from build123d import *

# Parameters (mm, degrees)
F0_W     = 25
F0_H     = 10
F1_DEPTH = 5
F2_R     = 1.4
F3_DEPTH = 25
F2_W     = 8
F2_H     = 10
F4_DEPTH = 7
F5_R     = 1.4
F6_DEPTH = 25
F2_R_2   = 2.5
F7_DEPTH = 2.5


with BuildPart() as f1:
    # F0 (on Top) → F1 (new body)
    with BuildSketch(Plane.XY):
        Rectangle(F0_W, F0_H)
    extrude(amount=F1_DEPTH)

    # F2 (on face) → F3 (cut)
    with BuildSketch(Plane.XY.offset(5)):
        with Locations((-9.5, 0.5)):
            Circle(F2_R)
    extrude(amount=-F3_DEPTH, mode=Mode.SUBTRACT)

    # F2 (on face) → F4 (join)
    with BuildSketch(Plane.XY.offset(5)):
        with Locations((8.5, 0)):
            Rectangle(F2_W, F2_H)
    extrude(amount=F4_DEPTH)

    # F5 (on face) → F6 (cut)
    with BuildSketch(Plane(origin=(4.5, 0, 0), x_dir=(0, -1, 0), z_dir=(-1, 0, 0))):
        with Locations((-2.647824, 9.4)):
            Circle(F5_R)
    extrude(amount=-F6_DEPTH, mode=Mode.SUBTRACT)

    # F2 (on face) → F7 (cut)
    with BuildSketch(Plane.XY.offset(5)):
        with Locations((-9.5, 0.5)):
            Circle(F2_R_2)
        with Locations((-9.5, 0.5)):
            Circle(F2_R, mode=Mode.SUBTRACT)
    extrude(amount=-F7_DEPTH, mode=Mode.SUBTRACT)


solid = f1.part
Geometry check sheet. Reference: the model listing, model coordinates, mm. A direction names the side the tool comes from. Round coordinates to 2 decimals unless told otherwise and drop trailing zeros. Write each loop counter-clockwise with the first axis right and the second up, starting at its lowest first coordinate (ties: lowest second). Pieces come first, ordered by that corner, then holes. Notation, with made-up numbers: (-39, -3) -> (-9, -3) arc R20 ccw to (-9, 32) -> close; hole circle Ø4 at (72, 84). An arc over 180 degrees is marked (long way). One line per item, written item: value. Start each with the question number.
(1) Cross-section at B-B, the plane z = 1.5. Record the cut outline in (x, y), and give its area (3 significant figures).
(2) Go/stop test with flat-tipped pins: pin 1 Ø4.5 at (y, z) = (2.65, 9.4) entering from -X; pin 2 Ø2 at (x, y) = (-9.5, 0.5) entering from +Z; pin 3 Ø5.5 at (x, y) = (-9.5, 1) entering from +Z. Record where each tip stops, or that it passes through.
(3) Cross-section at C-C, the plane x = 7.5. Record the cut outline in (y, z).
(4) Draft check along Y on faces 4 (the cylindrical face through (8.444, 1.312, 9.821)), 5 (the flat face through (12.5, 0, 6)), 6 (the flat face through (2.6, 5, 4.6)). Enter one of: +Y half, -Y half, draft (parallel to the pull), parting line (faces both ways), or undercut.
(5) Scan lines: line 1 (Y direction, x = -9.5, z = 4.3); line 2 (X direction, y = 4, z = 8.5); line 3 (Z direction, x = 3.5, y = 1). Record each from-to range of solid material in increasing order. Write a range as [from, to].
(6) Cross-section at D-D, the plane z = 9.4. Record the cut outline in (x, y).
(7) Cross-section at A-A, the plane y = 0.5. Record the cut outline in (x, z), and give its area (4 significant figures).
(8) Access from +Z, -Z, +X, -X, +Y, -Y to the whole of each face (thin tool, end or side, straight path). Record for faces 1 (the flat face through (-4, 0, 5)), 2 (the flat face through (-8, -1, 2.5)), 3 (the flat face through (8, 0, 12)).
Answer:
1. outline: (-12.5, -5) -> (12.5, -5) -> (12.5, 5) -> (-12.5, 5) -> close; hole circle Ø2.8 at (-9.5, 0.5)
1. area: 244 mm²
2. pin 1: x = 4.5
2. pin 2: through
2. pin 3: z = 5
3. outline: (-5, 0) -> (5, 0) -> (5, 12) -> (-5, 12) -> close; hole circle Ø2.8 at (2.65, 9.4)
4. face 4: undercut
4. face 5: draft
4. face 6: +Y half
5. line 1: [-5, -2], [3, 5]
5. line 2: [4.5, 12.5]
5. line 3: [0, 5]
6. outline: (4.5, -5) -> (12.5, -5) -> (12.5, 1.25) -> (4.5, 1.25) -> close; (4.5, 4.05) -> (12.5, 4.05) -> (12.5, 5) -> (4.5, 5) -> close
7. outline: (-12.5, 0) -> (-10.9, 0) -> (-10.9, 2.5) -> (-12, 2.5) -> (-12, 5) -> (-12.5, 5) -> close; (-8.1, 0) -> (12.5, 0) -> (12.5, 12) -> (4.5, 12) -> (4.5, 5) -> (-7, 5) -> (-7, 2.5) -> (-8.1, 2.5) -> close
7. area: 161.5 mm²
8. face 1: +Z, -X, +Y, -Y
8. face 2: +Z
8. face 3: +Z, +X, -X, +Y, -Y
